Design review of the part built by this model. Coordinates are the model's own, in mm. Face numbers are marked on the shaded views. A direction names the side the tool comes from. Give positions to 0.01 mm unless a question says otherwise; leave off trailing zeros. Loops run counter-clockwise (first coordinate to the right, second up) from the corner with the lowest first, then second, coordinate; pieces in that order, holes last. Notation, with made-up numbers: M -9.75,17 L 48.25,17 A19 cw 48.25,44 Z; hole C 84.5,75 d10. An arc over 180 degrees is marked long. Use one line per item in the form item = value. Start each with the question number.
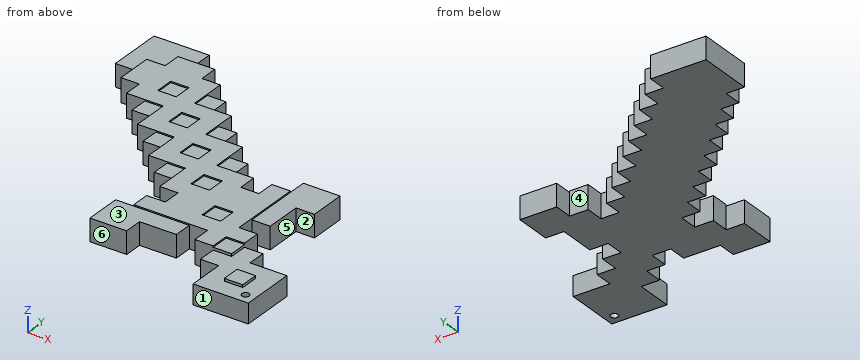
from build123d import *

# Parameters (mm, degrees)
F0_W     = 17.78
F0_H     = 17.78
F0_W_2   = 35.56
F0_W_3   = 17.9974469995
F0_H_2   = 35.56
F1_DEPTH = 19.05
F2_DEPTH = 21.59
F3_DEPTH = 3.81
F4_D     = 7.1374


with BuildPart() as f1:
    # F0 (on Top) → F1 (new body)
    with BuildSketch(Plane.XY):
        Polygon((-134.7540525866, 124.46), (-134.7540525866, 124.2569237947), (-117.5547838211, 124.2569237947), (-117.5547838211, 142.24), (-134.7540525866, 142.24), align=None)
        with Locations((-161.4240525866, 151.13)):
            Rectangle(F0_W, F0_H)
        with Locations((-63.6340525866, 26.67)):
            Rectangle(F0_W_2, F0_H)
        with Locations((-179.2040525866, 168.91)):
            Rectangle(F0_W, F0_H)
        with Locations((-90.3040525866, 133.35)):
            Rectangle(F0_W, F0_H)
        Polygon((-10.2940525866, 106.68), (-10.2940525866, 88.9), (7.4859474134, 88.9), (7.4859474134, 106.7038958168), (-10.2940525866, 106.7038958168), align=None)
        with Locations((-72.5240525866, 97.79)):
            Rectangle(F0_W, F0_H)
        with Locations((16.3759474134, -8.89)):
            Rectangle(F0_W, F0_H)
        with Locations((-90.4127760863, 26.67)):
            Rectangle(F0_W_3, F0_H)
        with Locations((-72.5240525866, 115.57)):
            Rectangle(F0_W, F0_H)
        with Locations((-19.1840525866, 44.45)):
            Rectangle(F0_W, F0_H)
        with Locations((-143.6440525866, 151.13)):
            Rectangle(F0_W, F0_H)
        with Locations((-143.6440525866, 186.69)):
            Rectangle(F0_W, F0_H)
        with Locations((-108.0840525866, 151.13)):
            Rectangle(F0_W, F0_H)
        with Locations((-1.4040525866, -8.89)):
            Rectangle(F0_W, F0_H)
        Polygon((60.8259474134, 0), (25.2659474134, 0), (25.2659474134, -17.78), (7.4859474134, -17.78), (7.4859474134, -53.34), (60.8259474134, -53.34), align=None)
        with Locations((34.1559474134, -26.67)):
            Rectangle(F0_W, F0_H, mode=Mode.SUBTRACT)
        with Locations((-161.4240525866, 133.35)):
            Rectangle(F0_W, F0_H)
        with Locations((-108.0840525866, 115.57)):
            Rectangle(F0_W, F0_H)
        Polygon((-28.0740525866, 0), (-10.2940525866, 0), (-10.2940525866, 17.78), (7.4859474134, 17.78), (7.4859474134, 35.56), (-10.1443827152, 35.56), (-10.1443827152, 17.9467629641), (-28.0740525866, 17.9467629641), (-28.0740525866, 17.78), align=None)
        with Locations((-90.3040525866, 62.23)):
            Rectangle(F0_W, F0_H)
        with Locations((-161.4240525866, 204.47)):
            Rectangle(F0_W, F0_H)
        Polygon((-10.1443827152, 17.9467629641), (-10.1443827152, 35.56), (-10.2940525866, 35.56), (-28.0740525866, 35.56), (-28.0740525866, 17.9467629641), align=None)
        with Locations((-54.7440525866, 80.01)):
            Rectangle(F0_W, F0_H)
        with Locations((-196.9840525866, 168.91)):
            Rectangle(F0_W, F0_H)
        with Locations((-143.6440525866, 168.91)):
            Rectangle(F0_W, F0_H)
        with Locations((-108.0840525866, 80.01)):
            Rectangle(F0_W, F0_H)
        with Locations((-161.4240525866, 168.91)):
            Rectangle(F0_W, F0_H)
        with Locations((-179.2040525866, 186.69)):
            Rectangle(F0_W, F0_H)
        with Locations((-143.6440525866, 133.35)):
            Rectangle(F0_W, F0_H)
        with Locations((-90.4127760863, 8.89)):
            Rectangle(F0_W_3, F0_H)
        Polygon((-45.8540525866, 17.78), (-28.0740525866, 17.78), (-28.0740525866, 17.9467629641), (-28.0740525866, 35.56), (-45.8540525866, 35.56), align=None)
        with Locations((-54.7440525866, 97.79)):
            Rectangle(F0_W, F0_H)
        with Locations((-72.5240525866, 62.23)):
            Rectangle(F0_W, F0_H)
        with Locations((-196.9840525866, 204.47)):
            Rectangle(F0_W, F0_H)
        with Locations((34.1559474134, -26.67)):
            Rectangle(F0_W, F0_H)
        with Locations((-63.6340525866, 8.89)):
            Rectangle(F0_W_2, F0_H)
        with Locations((-214.7640525866, 222.25)):
            Rectangle(F0_W, F0_H)
        with Locations((-72.5240525866, 80.01)):
            Rectangle(F0_W, F0_H)
        with Locations((-179.2040525866, 222.25)):
            Rectangle(F0_W, F0_H)
        Polygon((-152.5340525866, 106.68), (-134.7540525866, 106.68), (-134.7540525866, 124.2569237947), (-134.7540525866, 124.46), (-152.5340525866, 124.46), align=None)
        with Locations((-161.4240525866, 186.69)):
            Rectangle(F0_W, F0_H)
        with Locations((-1.4040525866, 71.12)):
            Rectangle(F0_W, F0_H_2)
        with Locations((-125.8640525866, 97.79)):
            Rectangle(F0_W, F0_H)
        with Locations((-90.3040525866, 115.57)):
            Rectangle(F0_W, F0_H)
        with Locations((-1.4040525866, 8.89)):
            Rectangle(F0_W, F0_H)
        with Locations((-90.3040525866, 97.79)):
            Rectangle(F0_W, F0_H)
        Polygon((-99.4114995861, 0), (-99.4114995861, 17.78), (-116.9740525866, 17.78), (-116.9740525866, -17.78), (-81.4140525866, -17.78), (-81.4140525866, 0), align=None)
        Polygon((-28.0740525866, 88.9), (-10.2940525866, 88.9), (-10.2940525866, 106.68), (-28.2914995861, 106.68), (-28.2914995861, 88.9), align=None)
        with Locations((-196.9840525866, 222.25)):
            Rectangle(F0_W, F0_H)
        with Locations((-125.8640525866, 168.91)):
            Rectangle(F0_W, F0_H)
        Polygon((-241.4340525866, 195.58), (-223.6540525866, 195.58), (-223.6540525866, 213.36), (-223.6540525866, 231.14), (-205.8740525866, 231.14), (-188.0940525866, 231.14), (-188.0940525866, 248.92), (-223.6540525866, 248.92), (-241.4340525866, 248.92), (-241.4340525866, 231.14), align=None)
        with Locations((-90.3040525866, 80.01)):
            Rectangle(F0_W, F0_H)
        with Locations((-214.7640525866, 204.47)):
            Rectangle(F0_W, F0_H)
        with Locations((-179.2040525866, 204.47)):
            Rectangle(F0_W, F0_H)
        with Locations((-108.0840525866, 97.79)):
            Rectangle(F0_W, F0_H)
        with Locations((-179.2040525866, 151.13)):
            Rectangle(F0_W, F0_H)
        Polygon((7.4859474134, 106.7038958168), (7.4859474134, 88.9), (25.2659474134, 88.9), (25.2659474134, 124.46), (-10.2940525866, 124.46), (-10.2940525866, 106.7038958168), align=None)
        with Locations((-54.7440525866, 62.23)):
            Rectangle(F0_W, F0_H)
        with Locations((-196.9840525866, 186.69)):
            Rectangle(F0_W, F0_H)
        with Locations((-36.9640525866, 44.45)):
            Rectangle(F0_W, F0_H)
        Polygon((-81.4140525866, 35.56), (-45.8540525866, 35.56), (-45.8540525866, 53.34), (-63.6340525866, 53.34), (-81.4140525866, 53.34), align=None)
        Polygon((-45.8540525866, 53.34), (-28.0740525866, 53.34), (-28.0740525866, 88.9), (-28.2914995861, 88.9), (-45.8540525866, 88.9), (-45.8540525866, 71.12), align=None)
        with Locations((-19.1840525866, 71.12)):
            Rectangle(F0_W, F0_H_2)
        Polygon((-117.5547838211, 142.24), (-116.9740525866, 142.24), (-116.9740525866, 160.02), (-134.7540525866, 160.02), (-134.7540525866, 142.24), align=None)
        Polygon((-134.7540525866, 106.68), (-116.9740525866, 106.68), (-116.9740525866, 124.46), (-99.1940525866, 124.46), (-99.1940525866, 142.24), (-116.9740525866, 142.24), (-117.5547838211, 142.24), (-117.5547838211, 124.2569237947), (-134.7540525866, 124.2569237947), align=None)
        with Locations((16.3759474134, 8.89)):
            Rectangle(F0_W, F0_H)
        with Locations((-214.7640525866, 186.69)):
            Rectangle(F0_W, F0_H)
    extrude(amount=F1_DEPTH)

    # F0 (on Top) → F2 (join)
    with BuildSketch(Plane.XY):
        with Locations((34.1559474134, -26.67)):
            Rectangle(F0_W, F0_H)
        with Locations((-1.4040525866, 8.89)):
            Rectangle(F0_W, F0_H)
        with Locations((-36.9640525866, 44.45)):
            Rectangle(F0_W, F0_H)
        Polygon((-10.2940525866, 106.68), (-10.2940525866, 88.9), (7.4859474134, 88.9), (7.4859474134, 106.7038958168), (-10.2940525866, 106.7038958168), align=None)
        Polygon((7.4859474134, 106.7038958168), (7.4859474134, 88.9), (25.2659474134, 88.9), (25.2659474134, 124.46), (-10.2940525866, 124.46), (-10.2940525866, 106.7038958168), align=None)
        with Locations((-1.4040525866, 71.12)):
            Rectangle(F0_W, F0_H_2)
        with Locations((-63.6340525866, 8.89)):
            Rectangle(F0_W_2, F0_H)
        Polygon((-99.4114995861, 0), (-99.4114995861, 17.78), (-116.9740525866, 17.78), (-116.9740525866, -17.78), (-81.4140525866, -17.78), (-81.4140525866, 0), align=None)
        with Locations((-90.4127760863, 8.89)):
            Rectangle(F0_W_3, F0_H)
        with Locations((-72.5240525866, 80.01)):
            Rectangle(F0_W, F0_H)
        with Locations((-108.0840525866, 115.57)):
            Rectangle(F0_W, F0_H)
        with Locations((-143.6440525866, 151.13)):
            Rectangle(F0_W, F0_H)
        with Locations((-179.2040525866, 186.69)):
            Rectangle(F0_W, F0_H)
        with Locations((-214.7640525866, 222.25)):
            Rectangle(F0_W, F0_H)
        Polygon((-241.4340525866, 195.58), (-223.6540525866, 195.58), (-223.6540525866, 213.36), (-223.6540525866, 231.14), (-205.8740525866, 231.14), (-188.0940525866, 231.14), (-188.0940525866, 248.92), (-223.6540525866, 248.92), (-241.4340525866, 248.92), (-241.4340525866, 231.14), align=None)
        with Locations((-143.6440525866, 186.69)):
            Rectangle(F0_W, F0_H)
        with Locations((-179.2040525866, 151.13)):
            Rectangle(F0_W, F0_H)
        with Locations((-108.0840525866, 151.13)):
            Rectangle(F0_W, F0_H)
        Polygon((-152.5340525866, 106.68), (-134.7540525866, 106.68), (-134.7540525866, 124.2569237947), (-134.7540525866, 124.46), (-152.5340525866, 124.46), align=None)
        with Locations((-72.5240525866, 115.57)):
            Rectangle(F0_W, F0_H)
        with Locations((-108.0840525866, 80.01)):
            Rectangle(F0_W, F0_H)
    extrude(amount=F2_DEPTH)

    # F3 (add): a face of the model
    f3_faces = [f1.faces().sort_by_distance(p)[0] for p in [
        (-90.3040525866, 138.9711867719, 19.05),
    ]]
    extrude(f3_faces, amount=F3_DEPTH)

    # F4 (through all)
    with Locations(Plane(origin=(0, 0, 0), x_dir=(1, 0, 0), z_dir=(0, 0, -1))):
        with Locations((51.5112578869, 43.6358898878)):
            Hole(F4_D / 2)


solid = f1.part
Q1. Take a section at B-B on y = 10. Give the boundary of the cut face in (x, z).
Q2. Take a section at D-D on y = 45.5. Give the boundary of the cut face in (x, z), plus the area to 3 significant figures.
Q3. Wall thickness on probe 1 along Y at (x, z) = (-116, 18.5); probe 2 along X at (y, z) = (11.5, 6.25); probe 3 along X at (y, z) = (118.5, 5.25): over which ranges is each line inside the solid? List them lowest first.
Q4. Take a section at C-C on x = -40. Give the boundary of the cut face in (y, z), plus the area to 3 significant figures.
Q5. For the marked faces 4, 5 and 6, list the 3-axis set-ups (+Z, -Z, +X, -X, +Y, -Y) from which the entire face can be reached by the end or side of a thin tool; tool diameter is ignored.
Q6. Clearance check with flat-ended pins moving along their axes: pin 1 Ø10 at (x, z) = (26, 8) entering from +Y; pin 2 Ø11.5 at (y, z) = (196.5, 16.5) entering from +X; pin 3 Ø5.5 at (y, z) = (155, 15.5) entering from -X; pin 4 Ø10 at (x, y) = (-152, 197.5) entering from -Z. State where each tip first meets the part, or that it passes through.
Q7. The part is to be moulded in two halves that separate along Y. For the marked faces 1, 2 and 3, say which applies: pulls with the +Y half, pulls with the -Y half, needs draft (parallel to the pull), parting line crosses it, or undercut.
Q8. Take a section at A-A on x = 1. Give the boundary of the cut face in (y, z), plus the area to 3 significant figures.
Response values:
q1.outline = M -116.97,0 L -45.85,0 L -45.85,21.59 L -116.97,21.59 Z; M -28.07,0 L 25.27,0 L 25.27,19.05 L 7.49,19.05 L 7.49,21.59 L -10.29,21.59 L -10.29,22.86 L -28.07,22.86 Z
q2.outline = M -81.41,0 L -10.29,0 L -10.29,22.86 L -28.07,22.86 L -28.07,21.59 L -45.85,21.59 L -45.85,22.86 L -81.41,22.86 Z
q2.area = 1,600 mm^2
q3.probe_1 = -17.78 to 17.78, 71.12 to 160.02
q3.probe_2 = -116.97 to -45.85, -28.07 to 25.27
q3.probe_3 = -152.53 to -63.63, -10.29 to 25.27
q4.outline = M 17.78,0 L 88.9,0 L 88.9,22.86 L 53.34,22.86 L 53.34,21.59 L 35.56,21.59 L 35.56,22.86 L 17.78,22.86 Z
q4.area = 1,600 mm^2
q5.face_4 = +Z, -Z, +Y
q5.face_5 = +Z, -Z, +X
q5.face_6 = +Z, -Z, -X, -Y
q6.pin_1 = 124.46
q6.pin_2 = -134.75
q6.pin_3 = -188.09
q6.pin_4 = 0
q7.face_1 = pulls with the -Y half
q7.face_2 = undercut
q7.face_3 = needs draft
q8.outline = M -17.78,0 L 35.56,0 L 35.56,22.86 L 17.78,22.86 L 17.78,21.59 L 0,21.59 L 0,19.05 L -17.78,19.05 Z; M 53.34,0 L 124.46,0 L 124.46,21.59 L 53.34,21.59 Z
q8.area = 2,660 mm^2
